from build123d import *

# Parameters (mm, degrees)
CROQUIS1_W              = 38.1
CROQUIS1_H              = 850.5
SALIENTE_EXTRUIR1_DEPTH = 6.31
CROQUIS2_W              = 38.1
CROQUIS2_H              = 6.31
SALIENTE_EXTRUIR2_DEPTH = 70
CROQUIS3_W              = 38.1
CROQUIS3_H              = 6.31
SALIENTE_EXTRUIR3_DEPTH = 578
CROQUIS4_R              = 6.935856655
CORTAR_EXTRUIR1_DEPTH   = 7
CROQUIS5_W              = 38.1
CROQUIS5_H              = 687.72607772
CORTAR_EXTRUIR2_DEPTH   = 10
CROQUIS6_W              = 38.1
CROQUIS6_H              = 6.31
CROQUIS8_W              = 368.89
CROQUIS8_H              = 6.31
CORTAR_EXTRUIR3_DEPTH   = 147
CROQUIS9_R              = 6.35
CORTAR_EXTRUIR4_DEPTH   = 6.31


with BuildPart() as part:
    # Croquis1 → Saliente-Extruir1 (new body)
    with BuildSketch(Plane.XY):
        Rectangle(CROQUIS1_W, CROQUIS1_H)
    extrude(amount=SALIENTE_EXTRUIR1_DEPTH)

    # Croquis2 → Saliente-Extruir2 (add)
    with BuildSketch(Plane.XY.offset(6.31)):
        with Locations((0, -422.095)):
            Rectangle(CROQUIS2_W, CROQUIS2_H)
    extrude(amount=SALIENTE_EXTRUIR2_DEPTH)

    # Croquis3 → Saliente-Extruir3 (add)
    with BuildSketch(Plane.XY.offset(6.31)):
        with Locations((0, -265.63107772)):
            Rectangle(CROQUIS3_W, CROQUIS3_H)
    extrude(amount=-SALIENTE_EXTRUIR3_DEPTH)

    # Croquis4 → Cortar-Extruir1 (cut)
    with BuildSketch(Plane(origin=(0, -262.47607772, 0), x_dir=(1, 0, 0), z_dir=(0, 1, 0))):
        with Locations(Location((0, 536.981534281, 0), (0, 0, 270))):
            Circle(CROQUIS4_R)
    extrude(amount=-CORTAR_EXTRUIR1_DEPTH, mode=Mode.SUBTRACT)

    # Croquis5 → Cortar-Extruir2 (cut)
    with BuildSketch(Plane(origin=(0, 0, 0), x_dir=(-1, 0, 0), z_dir=(0, 0, -1))):
        with Locations((0, 81.38696114)):
            Rectangle(CROQUIS5_W, CROQUIS5_H)
    extrude(amount=-CORTAR_EXTRUIR2_DEPTH, mode=Mode.SUBTRACT)

    # Barrer1: sweep along a curve in space
    with BuildLine() as barrer1_path:
        Line((0, -262.47607772, -199.645), (0, 386.85392228, -199.645))
        Line((0, 386.85392228, -199.645), (0, 386.85392228, 127.905))
    # Croquis6 → Barrer1 (sweep)
    with BuildSketch(Plane(origin=(0, -262.47607772, 0), x_dir=(1, 0, 0), z_dir=(0, 1, 0))):
        with Locations((0, 199.645)):
            Rectangle(CROQUIS6_W, CROQUIS6_H)
    sweep(path=barrer1_path.line, transition=Transition.RIGHT)

    # Croquis8 → Cortar-Extruir3 (cut)
    with BuildSketch(Plane(origin=(19.05, 0, 0), x_dir=(0, 0, -1), z_dir=(1, 0, 0))):
        Polygon((196.49, -262.47607772), (196.49, -268.78607772), (196.49, -444.307673596), (-90.834600665, -444.307673596), (-90.834600665, -262.47607772), align=None)
        with Locations((387.245, -265.63107772)):
            Rectangle(CROQUIS8_W, CROQUIS8_H)
    extrude(amount=-CORTAR_EXTRUIR3_DEPTH, mode=Mode.SUBTRACT)

    # Croquis9 → Cortar-Extruir4 (cut)
    with BuildSketch(Plane(origin=(0, 390.00892228, 0), x_dir=(1, 0, 0), z_dir=(0, 1, 0))):
        with Locations(Location((0, -84.010000001, 0), (0, 0, 180))):
            Circle(CROQUIS9_R)
        with Locations(Location((0, -116.010000001, 0), (0, 0, 180))):
            Circle(CROQUIS9_R)
    extrude(amount=-CORTAR_EXTRUIR4_DEPTH, mode=Mode.SUBTRACT)


solid = part.part
Here's how the part is built. I have some questions about the finished solid (model axes, mm). Coordinates: 2 decimals unless noted, no trailing zeros. Loops run counter-clockwise (first coordinate to the right, second up) from the corner with the lowest first, then second, coordinate; pieces in that order, holes last.
1. Imagine slicing it at D-D, the plane y = 43. Please give me the cut outline in (x, z).
2. If we mould it in two halves opening along Z, with no side actions, what happens to faces 1 (the cylindrical face through (1.38, 386.9, 77.81)), 2 (the flat face through (0, 53, -196.49)), 3 (the cylindrical face through (1.38, 386.9, 109.81)), 4 (the flat face through (0, 383.699, -32))? For each: pulls with the +Z half, pulls with the -Z half, needs draft (parallel to the pull), parting line crosses it, or undercut.
3. Imagine slicing it at C-C, the plane z = 8.5. Please give me the cut outline in (x, y), and give its area (3 significant figures).
4. Imagine slicing it at B-B, the plane x = 0. Please give me the cut outline in (y, z) (3 decimals), and give its area (3 significant figures).
5. For P1, Ø10, axis at x = 3, y = 213.5, coming from the +Z side; P2, Ø11.5, axis at x = -5, z = -18.5, coming from the -Y side, each with a flat end and sliding along its axis, tell me the tip position at first contact or that it passes through.
6. I need wall thicknesses on L1, parallel to Z at x = 0, y = 388 (3 decimals); L2, parallel to X at y = 386, z = 116; L3, parallel to Y at x = -6, z = 78. Which ranges of each line are inside material? Lowest first, please.
7. Imagine slicing it at A-A, the plane z = 84.01. Please give me the cut outline in (x, y).
Taken from the geometry:
1. outline: (-19.05, -202.8) - (19.05, -202.8) - (19.05, -196.49) - (-19.05, -196.49) - close
2. face 1: undercut
2. face 2: pulls with the +Z half
2. face 3: undercut
2. face 4: needs draft
3. outline: (-19.05, 383.7) - (19.05, 383.7) - (19.05, 390.01) - (-19.05, 390.01) - close
3. area: 240 mm2
4. outline: (-268.786, -202.8) - (390.009, -202.8) - (390.009, 77.66) - (383.699, 77.66) - (383.699, -196.49) - (-268.786, -196.49) - close; (383.699, 90.36) - (390.009, 90.36) - (390.009, 109.66) - (383.699, 109.66) - close; (383.699, 122.36) - (390.009, 122.36) - (390.009, 127.905) - (383.699, 127.905) - close
4. area: 6,040 mm2
5. P1: stops at z = -196.49
5. P2: stops at y = 383.7
6. L1: z = -202.8 to 77.66, 90.36 to 109.66, 122.36 to 127.905
6. L2: x = -19.05 to -6.35, 6.35 to 19.05
6. L3: y = 383.7 to 390.01
7. outline: (-19.05, 383.7) - (-6.35, 383.7) - (-6.35, 390.01) - (-19.05, 390.01) - close; (6.35, 383.7) - (19.05, 383.7) - (19.05, 390.01) - (6.35, 390.01) - close
